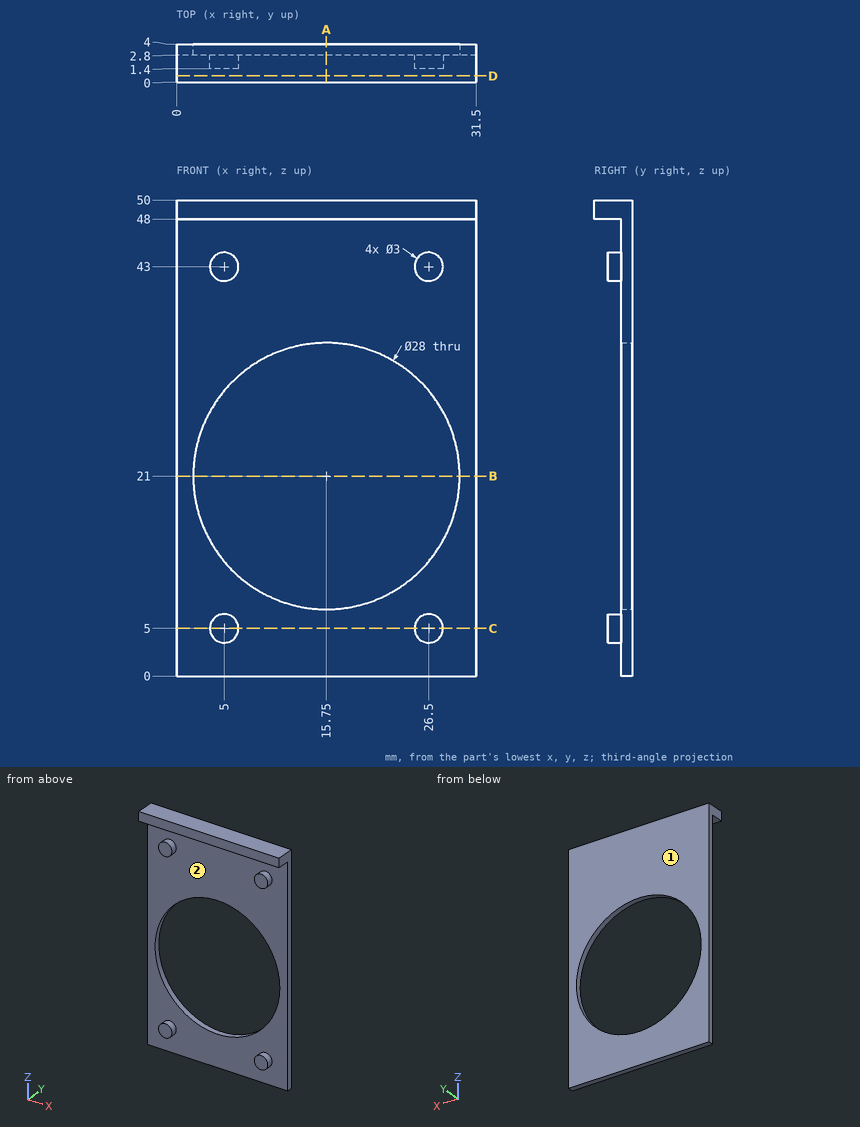
Design review of the part shown in the three views and the two pictorial views. Dimensions are in mm from the part's minimum x, y and z. Coordinates: 2 decimals unless noted, no trailing zeros. Loops run counter-clockwise (first coordinate to the right, second up) from the corner with the lowest first, then second, coordinate; pieces in that order, holes last.
(1) Draft analysis for pull direction Z (two halves, no side actions). For the marked faces 1 and 2, state which applies: +Z half, -Z half, draft (parallel to the pull), parting line (faces both ways), or undercut.
Determined:
face 1: draft
face 2: undercut
(2) Wall thickness on L1, parallel to Y at x = 4.5, z = 32.5; L2, parallel to Z at x = 15.75, y = 3.6; L3, parallel to X at y = 1.95, z = 6: over which ranges is each line inside the solid? List them lowest first.
Determined:
L1: y = 2.8 to 4
L2: z = 0 to 7, 35 to 50
L3: x = 3.88 to 6.12, 25.38 to 27.62
(3) Insertion check: P1, Ø1.5, axis at x = 4.5, z = 5, coming from the -Y side; P2, Ø12, axis at x = 25, z = 17, coming from the +Y side. Each pin has a flat end and moves straight along its axis. Give the tip position at first contact, or say it passes through.
Determined:
P1: stops at y = 1.4
P2: stops at y = 4
(4) Consider section D-D, the plane y = 0.65. Give the boundary of the cut face in (x, z), plus the area to 3 significant figures.
Determined:
outline: (0, 48) - (31.5, 48) - (31.5, 50) - (0, 50) - close
area: 63.0 mm2
(5) Consider section A-A, the plane x = 15.75. Give the boundary of the cut face in (y, z), plus the area to 3 significant figures.
Determined:
outline: (0, 48) - (2.8, 48) - (2.8, 35) - (4, 35) - (4, 50) - (0, 50) - close; (2.8, 0) - (4, 0) - (4, 7) - (2.8, 7) - close
area: 32.0 mm2
(6) Consider section B-B, the plane z = 21. Give the boundary of the cut face in (x, y).
Determined:
outline: (0, 2.8) - (1.75, 2.8) - (1.75, 4) - (0, 4) - close; (29.75, 2.8) - (31.5, 2.8) - (31.5, 4) - (29.75, 4) - close
(7) Consider section C-C, the plane z = 5. Give the boundary of the cut face in (x, y).
Determined:
outline: (0, 2.8) - (3.5, 2.8) - (3.5, 1.4) - (6.5, 1.4) - (6.5, 2.8) - (25, 2.8) - (25, 1.4) - (28, 1.4) - (28, 2.8) - (31.5, 2.8) - (31.5, 4) - (0, 4) - close
